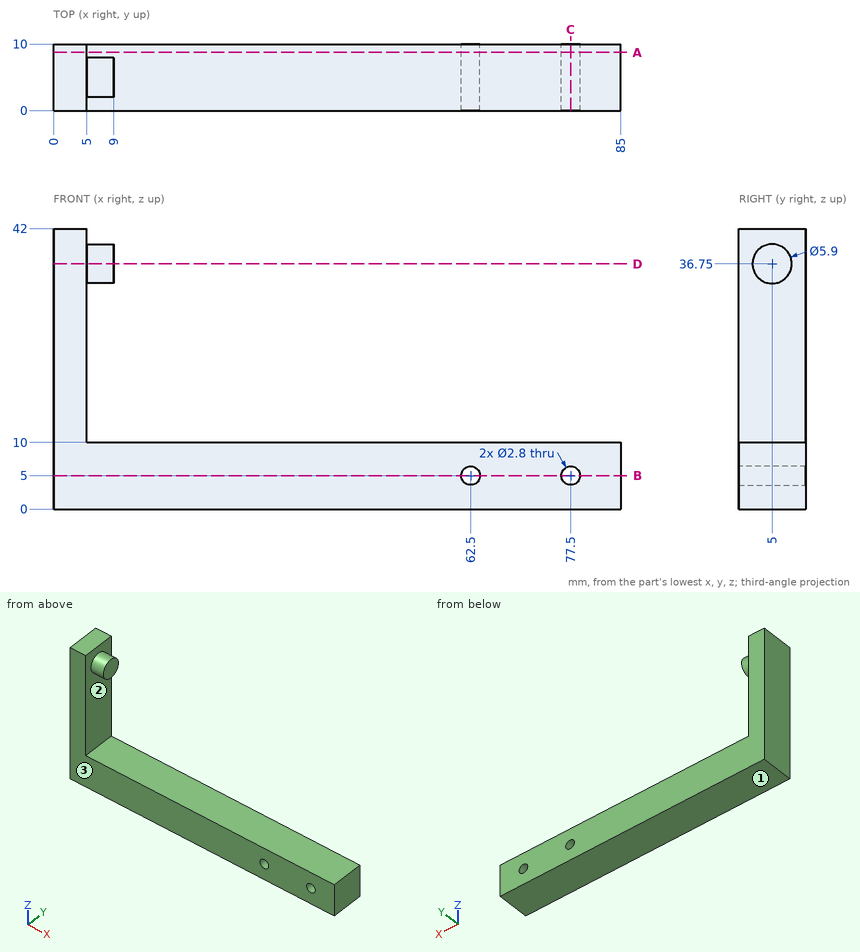
Geometry check sheet. Reference: drawing and pictorial views, mm from the part's lowest x, y, z. Coordinates: 2 decimals unless noted, no trailing zeros. Loops run counter-clockwise (first coordinate to the right, second up) from the corner with the lowest first, then second, coordinate; pieces in that order, holes last. Notation, with made-up numbers: (26.5, 4.25) -> (36.5, 4.25) arc R24 ccw to (36.5, 17.25) -> close; hole circle Ø9 at (6.25, -34). An arc over 180 degrees is marked (long way). Write item = value, one per line. Start each with the question number.
1. Section check C-C on x = 77.5. Record the cut outline in (y, z).
2. Section check B-B on z = 5. Record the cut outline in (x, y).
3. Draft check along Z on the marked faces 1, 2 and 3. Enter one of: released by +Z, released by -Z, zero draft, split by the parting line, or undercut.
4. Section check D-D on z = 36.75. Record the cut outline in (x, y).
5. Section check A-A on y = 8.75. Record the cut outline in (x, z).
6. Depth check by flat-ended pin: P1, Ø4, axis at y = 5, z = 29.5, coming from the -X side; P2, Ø1.7, axis at x = 62.5, z = 5, coming from the +Y side; P3, Ø5, axis at x = 69, y = 2, coming from the +Z side; P4, Ø4.5, axis at y = 4.5, z = 37, coming from the +X side. Enter the tip coordinate at first touch or a pass-through.
7. Material ranges on line 1 (Z direction, x = 77.5, y = 8); line 2 (X direction, y = 8.25, z = 4.5); line 3 (Z direction, x = 70.5, y = 4.75), recorded low to high.
Responses:
q1.outline = (0, 0) -> (10, 0) -> (10, 3.6) -> (0, 3.6) -> close; (0, 6.4) -> (10, 6.4) -> (10, 10) -> (0, 10) -> close
q2.outline = (0, 0) -> (61.1, 0) -> (61.1, 10) -> (0, 10) -> close; (63.9, 0) -> (76.1, 0) -> (76.1, 10) -> (63.9, 10) -> close; (78.9, 0) -> (85, 0) -> (85, 10) -> (78.9, 10) -> close
q3.face_1 = released by -Z
q3.face_2 = undercut
q3.face_3 = zero draft
q4.outline = (0, 0) -> (5, 0) -> (5, 2.05) -> (9, 2.05) -> (9, 7.95) -> (5, 7.95) -> (5, 10) -> (0, 10) -> close
q5.outline = (0, 0) -> (85, 0) -> (85, 10) -> (5, 10) -> (5, 42) -> (0, 42) -> close; hole circle Ø2.8 at (62.5, 5); hole circle Ø2.8 at (77.5, 5)
q6.P1 = 0
q6.P2 = through
q6.P3 = 10
q6.P4 = 9
q7.line_1 = 0 to 3.6, 6.4 to 10
q7.line_2 = 0 to 61.19, 63.81 to 76.19, 78.81 to 85
q7.line_3 = 0 to 10
